from build123d import *

# Parameters (mm, degrees)
SKETCH1_W            = 64.77
SKETCH1_H            = 50.546
SKETCH1_W_2          = 58.674
SKETCH1_H_2          = 40.386
BOSS_EXTRUDE1_DEPTH  = 12.7
BOSS_EXTRUDE2_DEPTH  = 2.54
BOSS_EXTRUDE3_DEPTH  = 21.7932
SKETCH6_W            = 22.86
SKETCH6_H            = 2.667
SKETCH6_H_2          = 5.08
CUT_EXTRUDE1_DEPTH   = 102.661620763
SKETCH7_W            = 22.86
SKETCH7_H            = 5.08
SKETCH7_H_2          = 1.143
CUT_EXTRUDE2_DEPTH   = 12.7
SKETCH10_W           = 14.097
SKETCH10_H           = 6.35
BOSS_EXTRUDE4_DEPTH  = 5.08
BOSS_EXTRUDE5_DEPTH  = 3.81
SKETCH12_R           = 1.27
CUT_EXTRUDE3_DEPTH   = 109.200389682
BOSS_EXTRUDE7_DEPTH  = 3.81
SKETCH14_W           = 15.24
SKETCH14_H           = 6.35
BOSS_EXTRUDE8_DEPTH  = 5.08
SKETCH15_R           = 1.27
CUT_EXTRUDE4_DEPTH   = 113.497597873
BOSS_EXTRUDE9_DEPTH  = 3.81
BOSS_EXTRUDE10_DEPTH = 3.81


with BuildPart() as part:
    # Sketch1 → Boss-Extrude1 (new body)
    with BuildSketch(Plane.XY):
        Rectangle(SKETCH1_W, SKETCH1_H)
        Rectangle(SKETCH1_W_2, SKETCH1_H_2, mode=Mode.SUBTRACT)
    extrude(amount=BOSS_EXTRUDE1_DEPTH)

    # Sketch3 → Boss-Extrude2 (add)
    with BuildSketch(Plane.XY.offset(12.7)):
        Polygon((79.354012503, -25.273), (79.354012503, -22.098), (56.494012503, -22.098), (56.494012503, -25.273), (-32.385, -25.273), (-32.385, 26.797), (56.494012503, 26.797), (56.494012503, 24.257), (79.354012503, 24.257), (79.354012503, 26.797), (90.805, 26.797), (90.805, -25.273), align=None)
    extrude(amount=BOSS_EXTRUDE2_DEPTH)

    # Sketch5 → Boss-Extrude3 (add)
    with BuildSketch(Plane.XY.offset(15.24)):
        Polygon((-32.385, 26.797), (-32.385, -25.273), (56.494012503, -25.273), (56.494012503, -20.193), (-27.305, -20.193), (-27.305, 24.13), (56.494012503, 24.13), (56.494012503, 26.797), align=None)
        Polygon((79.354012503, -20.193), (79.354012503, -25.273), (90.805, -25.273), (90.805, 17.907), (88.011, 17.907), (88.011, -20.193), align=None)
    extrude(amount=BOSS_EXTRUDE3_DEPTH)

    # Sketch6 → Cut-Extrude1 (cut, through all)
    with BuildSketch(Plane.XY.offset(37.0332)):
        with Locations((3.175, 25.4635)):
            Rectangle(SKETCH6_W, SKETCH6_H)
        with Locations((3.175, -22.733)):
            Rectangle(SKETCH6_W, SKETCH6_H_2)
    extrude(amount=-CUT_EXTRUDE1_DEPTH, mode=Mode.SUBTRACT)

    # Sketch7 → Cut-Extrude2 (cut)
    with BuildSketch(Plane(origin=(0, 0, 0), x_dir=(-1, 0, 0), z_dir=(0, 0, -1))):
        with Locations((-3.175, 22.733)):
            Rectangle(SKETCH7_W, SKETCH7_H)
        with Locations((-3.175, -20.7645)):
            Rectangle(SKETCH7_W, SKETCH7_H_2)
    extrude(amount=-CUT_EXTRUDE2_DEPTH, mode=Mode.SUBTRACT)

    # Sketch10 → Boss-Extrude4 (add)
    with BuildSketch(Plane.ZY.offset(32.385)):
        with Locations((18.5166, -22.098)):
            Rectangle(SKETCH10_W, SKETCH10_H)
    extrude(amount=BOSS_EXTRUDE4_DEPTH)

    # Sketch11 → Boss-Extrude5 (add)
    with BuildSketch(Plane.XY.offset(25.5651)):
        Polygon((-37.465, -18.923), (-32.385, -18.923), (-32.385, -13.843), align=None)
    extrude(amount=-BOSS_EXTRUDE5_DEPTH)

    # Sketch12 → Cut-Extrude3 (cut, through all)
    with BuildSketch(Plane(origin=(0, -18.923, 0), x_dir=(1, 0, 0), z_dir=(0, 1, 0))):
        with Locations(Location((-34.925, -18.5166, 0), (0, 0, 270))):
            Circle(SKETCH12_R)
    extrude(amount=-CUT_EXTRUDE3_DEPTH, mode=Mode.SUBTRACT)

    # Sketch13 → Boss-Extrude7 (add)
    with BuildSketch(Plane(origin=(0, 0, 11.4681), x_dir=(-1, 0, 0), z_dir=(0, 0, -1))):
        Polygon((32.385, -13.843), (32.385, -18.923), (37.465, -18.923), align=None)
    extrude(amount=-BOSS_EXTRUDE7_DEPTH)

    # Sketch14 → Boss-Extrude8 (add)
    with BuildSketch(Plane(origin=(90.805, 0, 0), x_dir=(0, 0, -1), z_dir=(1, 0, 0))):
        with Locations((-24.8666, -22.098)):
            Rectangle(SKETCH14_W, SKETCH14_H)
    extrude(amount=BOSS_EXTRUDE8_DEPTH)

    # Sketch15 → Cut-Extrude4 (cut, through all)
    with BuildSketch(Plane(origin=(0, -18.923, 0), x_dir=(1, 0, 0), z_dir=(0, 1, 0))):
        with Locations(Location((93.345, -24.8666, 0), (0, 0, 270))):
            Circle(SKETCH15_R)
    extrude(amount=-CUT_EXTRUDE4_DEPTH, mode=Mode.SUBTRACT)

    # Sketch17 → Boss-Extrude9 (add)
    with BuildSketch(Plane.XY.offset(32.4866)):
        Polygon((95.885, -18.923), (90.805, -18.923), (90.805, -13.843), align=None)
    extrude(amount=-BOSS_EXTRUDE9_DEPTH)

    # Sketch18 → Boss-Extrude10 (add)
    with BuildSketch(Plane(origin=(0, 0, 17.2466), x_dir=(-1, 0, 0), z_dir=(0, 0, -1))):
        Polygon((-95.885, -18.923), (-90.805, -18.923), (-90.805, -13.843), align=None)
    extrude(amount=-BOSS_EXTRUDE10_DEPTH)


solid = part.part
Here's how the part is built. I have some questions about the finished solid (model axes, mm). A direction names the side the tool comes from. Round coordinates to 2 decimals unless told otherwise and drop trailing zeros. Loops run counter-clockwise (first coordinate to the right, second up) from the corner with the lowest first, then second, coordinate; pieces in that order, holes last. Notation, with made-up numbers: (82.5, 84) -> (117.5, 84) arc R24 cw to (117.5, 110) -> close; hole circle Ø10 at (64, 78.25). An arc over 180 degrees is marked (long way). Write each question's results on one line, items separated by ' | '.
(1) If I drill on L1, parallel to Y at x = -14, z = 12; L2, parallel to X at y = -5, z = 27.5 (3 decimals); L3, parallel to Y at x = 52, z = 29.5, over which ranges is the centre line in solid material (lowest first)?
Worked answers:
L1: -25.27 to -20.19, 20.19 to 25.27 | L2: -32.385 to -27.305, 88.011 to 90.805 | L3: -25.27 to -20.19, 24.13 to 26.8
(2) If we section it at D-D, the plane x = 25: List the corners of the cut face in (y, z) for me, then the cut area to 3 significant figures.
Worked answers:
outline: (-25.27, 0) -> (-20.19, 0) -> (-20.19, 12.7) -> (20.19, 12.7) -> (20.19, 0) -> (25.27, 0) -> (25.27, 12.7) -> (26.8, 12.7) -> (26.8, 37.03) -> (24.13, 37.03) -> (24.13, 15.24) -> (-20.19, 15.24) -> (-20.19, 37.03) -> (-25.27, 37.03) -> close | area: 430 mm2
(3) We'd pull the mould along X, two halves only. Please class faces 6 (the face through (-35, -21, 25.565)), 7 (the face through (32.385, 0, 6)), 8 (the face through (22, 20.193, 6)): released by +X, released by -X, zero draft, split by the parting line, or undercut.
Worked answers:
face 6: zero draft | face 7: released by +X | face 8: undercut
(4) For P1, Ø4, axis at y = -9, z = 26.5, coming from the -X side (3 decimals); P2, Ø8, axis at x = -7.5, y = 13.5, coming from the +Z side; P3, Ø1.4, axis at x = 89.5, z = 25.5, coming from the +Y side; P4, Ø14, axis at x = -20.5, z = 7, coming from the +Y side, each with a flat end and sliding along its axis, tell me the tip position at first contact or that it passes through.
Worked answers:
P1: x = -32.385 | P2: z = 15.24 | P3: y = 17.91 | P4: y = 26.8
(5) If we section it at C-C, the plane x = 40: List the corners of the cut face in (y, z) for me.
Worked answers:
outline: (-25.27, 12.7) -> (26.8, 12.7) -> (26.8, 37.03) -> (24.13, 37.03) -> (24.13, 15.24) -> (-20.19, 15.24) -> (-20.19, 37.03) -> (-25.27, 37.03) -> close
(6) For faces 1 (the face through (89, 17.907, 26)), 2 (the face through (-20, 25.273, 6)), 3 (the face through (-18, 24.13, 26)), 4 (the face through (85, 26.797, 14)), 5 (the face through (-18, -20.193, 26)), which set-ups out of +Z, -Z, +X, -X, +Y, -Y let a thin tool reach every point of the face, with its end or its side?
Worked answers:
face 1: +Z, +X, +Y | face 2: -Z, +X, -X, +Y | face 3: +Z, +X | face 4: +Z, -Z, +X, -X, +Y | face 5: +Z
(7) If we section it at A-A, the plane z = 8: List the corners of the cut face in (x, y) for me (3 decimals), then the cut area to 3 significant figures.
Worked answers:
outline: (-32.385, -25.273) -> (-8.255, -25.273) -> (-8.255, -20.193) -> (-29.337, -20.193) -> (-29.337, 20.193) -> (-8.255, 20.193) -> (-8.255, 25.273) -> (-32.385, 25.273) -> close; (14.605, -25.273) -> (32.385, -25.273) -> (32.385, 25.273) -> (14.605, 25.273) -> (14.605, 20.193) -> (29.337, 20.193) -> (29.337, -20.193) -> (14.605, -20.193) -> close | area: 672 mm2
(8) If we section it at B-B, the plane y = 0: List the corners of the cut face in (x, z) for me (3 decimals), then the cut area to 3 significant figures.
Worked answers:
outline: (-32.385, 0) -> (-29.337, 0) -> (-29.337, 12.7) -> (29.337, 12.7) -> (29.337, 0) -> (32.385, 0) -> (32.385, 12.7) -> (90.805, 12.7) -> (90.805, 37.033) -> (88.011, 37.033) -> (88.011, 15.24) -> (-27.305, 15.24) -> (-27.305, 37.033) -> (-32.385, 37.033) -> close | area: 562 mm2
